from build123d import *

# Parameters (mm, degrees)
BOSS_EXTRUDE1_DEPTH              = 1.6
BOSS_EXTRUDE2_DEPTH              = 0.1
M1_6_HOLE1_FIXINGSTRUCTURE_D     = 1.8
M1_6_HOLE1_FIXINGSTRUCTURE_DEPTH = 200
M1_6_HOLE1_FIXINGSTRUCTURE_TIP   = 0.540774557
SKETCH4_R                        = 1.1
CUT_EXTRUDE1_DEPTH               = 1.7


with BuildPart() as part:
    # Sketch1 → Boss-Extrude1 (new body)
    with BuildSketch(Plane.XY):
        with BuildLine():
            Line((-34, 44), (-34, 38))
            ThreePointArc((-34, 38), (-34.146446609, 37.646446609), (-34.5, 37.5))
            Line((-34.5, 37.5), (-40.5, 37.5))
            ThreePointArc((-40.5, 37.5), (-40.853553391, 37.353553391), (-41, 37))
            Line((-41, 37), (-41, -37))
            ThreePointArc((-41, -37), (-40.853553391, -37.353553391), (-40.5, -37.5))
            Line((-40.5, -37.5), (-34.5, -37.5))
            ThreePointArc((-34.5, -37.5), (-34.146446609, -37.646446609), (-34, -38))
            Line((-34, -38), (-34, -44))
            ThreePointArc((-34, -44), (-33.853553391, -44.353553391), (-33.5, -44.5))
            Line((-33.5, -44.5), (33.5, -44.5))
            ThreePointArc((33.5, -44.5), (33.853553391, -44.353553391), (34, -44))
            Line((34, -44), (34, -38))
            ThreePointArc((34, -38), (34.146446609, -37.646446609), (34.5, -37.5))
            Line((34.5, -37.5), (40.5, -37.5))
            ThreePointArc((40.5, -37.5), (40.853553391, -37.353553391), (41, -37))
            Line((41, -37), (41, 37))
            ThreePointArc((41, 37), (40.853553391, 37.353553391), (40.5, 37.5))
            Line((40.5, 37.5), (34.5, 37.5))
            ThreePointArc((34.5, 37.5), (34.146446609, 37.646446609), (34, 38))
            Line((34, 38), (34, 44))
            ThreePointArc((34, 44), (33.853553391, 44.353553391), (33.5, 44.5))
            Line((33.5, 44.5), (-33.5, 44.5))
            ThreePointArc((-33.5, 44.5), (-33.853553391, 44.353553391), (-34, 44))
        make_face()
    extrude(amount=BOSS_EXTRUDE1_DEPTH)

    # Esboço1 → Boss-Extrude2 (add)
    with BuildSketch(Plane.XY.offset(1.6)):
        with BuildLine():
            Line((-29.5, -37.5), (29.5, -37.5))
            ThreePointArc((29.5, -37.5), (33.035533906, -36.035533906), (34.5, -32.5))
            Line((34.5, -32.5), (34.5, 32.5))
            ThreePointArc((34.5, 32.5), (33.035533906, 36.035533906), (29.5, 37.5))
            Line((29.5, 37.5), (-29.5, 37.5))
            ThreePointArc((-29.5, 37.5), (-33.035533906, 36.035533906), (-34.5, 32.5))
            Line((-34.5, 32.5), (-34.5, -32.5))
            ThreePointArc((-34.5, -32.5), (-33.035533906, -36.035533906), (-29.5, -37.5))
        make_face()
    extrude(amount=BOSS_EXTRUDE2_DEPTH)

    # M1.6 Hole1-FixingStructure
    with Locations(Plane(origin=(0, 0, 0), x_dir=(-1, 0, 0), z_dir=(0, 0, -1))):
        with Locations((-30.5, 40.5), (30.5, 40.5), (-30.5, -40.5), (30.5, -40.5)):
            Hole(M1_6_HOLE1_FIXINGSTRUCTURE_D / 2, depth=M1_6_HOLE1_FIXINGSTRUCTURE_DEPTH)
            with Locations((0, 0, -(M1_6_HOLE1_FIXINGSTRUCTURE_DEPTH + M1_6_HOLE1_FIXINGSTRUCTURE_TIP / 2))):  # 118° drill point
                Cone(0, M1_6_HOLE1_FIXINGSTRUCTURE_D / 2, M1_6_HOLE1_FIXINGSTRUCTURE_TIP, mode=Mode.SUBTRACT)

    # Sketch4 → Cut-Extrude1 (cut)
    with BuildSketch(Plane.XY.offset(1.7)):
        with Locations((25.155444566, 1)):
            Circle(SKETCH4_R)
        with Locations((10, 27.25)):
            Circle(SKETCH4_R)
        with Locations((-5.155444566, 1)):
            Circle(SKETCH4_R)
    extrude(amount=-CUT_EXTRUDE1_DEPTH, mode=Mode.SUBTRACT)


solid = part.part
CAD build for the part. Positions are in the model's coordinates, mm. A direction names the side the tool comes from. Round coordinates to 2 decimals unless told otherwise and drop trailing zeros. Write each loop counter-clockwise with the first axis right and the second up, starting at its lowest first coordinate (ties: lowest second). Pieces come first, ordered by that corner, then holes.
(1) Slice it at B-B, the plane z = 0.4. Count the separate pieces of the cut face and the enclosed holes in it, and give its area (3 significant figures).
(2) Mould opens along Y. For faces 3 (the face through (-1, 1, 0)), 4 (the face through (-4.564, 1.928, 0.862)) say: pulls with the +Y half, pulls with the -Y half, needs draft (parallel to the pull), parting line crosses it, or undercut.
(3) Slice it at A-A, the plane y = 27.25. Write the cut outline in (x, z), and give its area (3 significant figures).
(4) Drop flat-ended pins along their axis: P1, Ø0.5, axis at y = 40.5, z = 1, coming from the +X side; P2, Ø2, axis at x = 30.5, y = -40.5, coming from the +Z side. Give the stop position or say it passes through.
(5) Slice it at D-D, the plane y = 1. Write the cut outline in (x, z), and give its area (3 significant figures).
(6) Probe line 1 along Y through (x, z) = (30.5, 0.65); line 2 along X through (y, z) = (40.5, 0.65); line 3 along X through (y, z) = (-40, 0.55). List the from-to ranges inside material, lowest first.
(7) 3-axis set-ups, long thin cutter, end or side, ignore diameter. For faces 1 (the face through (-37, 4, 1.6)), 2 (the face through (26.205, 1.33, 0.862)): which of +Z, -Z, +X, -X, +Y, -Y reach the whole face in a straight line?
(8) Slice it at C-C, the plane x = 10. Write the cut outline in (y, z).
From the geometry:
1. separate pieces: 1
1. enclosed holes: 7
1. area: 7,080 mm2
2. face 3: needs draft
2. face 4: undercut
3. outline: (-41, 0) - (8.9, 0) - (8.9, 1.7) - (-34.5, 1.7) - (-34.5, 1.6) - (-41, 1.6) - close; (11.1, 0) - (41, 0) - (41, 1.6) - (34.5, 1.6) - (34.5, 1.7) - (11.1, 1.7) - close
3. area: 134 mm2
4. P1: stops at x = 34
4. P2: stops at z = 1.6
5. outline: (-41, 0) - (-6.26, 0) - (-6.26, 1.7) - (-34.5, 1.7) - (-34.5, 1.6) - (-41, 1.6) - close; (-4.06, 0) - (24.06, 0) - (24.06, 1.7) - (-4.06, 1.7) - close; (26.26, 0) - (41, 0) - (41, 1.6) - (34.5, 1.6) - (34.5, 1.7) - (26.26, 1.7) - close
5. area: 131 mm2
6. line 1: y = -44.5 to -41.4, -39.6 to 39.6, 41.4 to 44.5
6. line 2: x = -34 to -31.4, -29.6 to 29.6, 31.4 to 34
6. line 3: x = -34 to -31.25, -29.75 to 29.75, 31.25 to 34
7. face 1: +Z
7. face 2: +Z, -Z
8. outline: (-44.5, 0) - (26.15, 0) - (26.15, 1.7) - (-37.5, 1.7) - (-37.5, 1.6) - (-44.5, 1.6) - close; (28.35, 0) - (44.5, 0) - (44.5, 1.6) - (37.5, 1.6) - (37.5, 1.7) - (28.35, 1.7) - close
